```python
from build123d import *

# Parameters (mm, degrees)
F0_W      = 18
F0_H      = 20
F0_R      = 2.5
F0_W_2    = 31
F0_H_2    = 18
F0_H_3    = 2
F1_DEPTH  = 5
F2_DEPTH  = 14
F3_W      = 16
F3_H      = 7
F5_W      = 16
F5_H      = 7
F7_DEPTH  = 0.25
F4_W      = 16
F4_H      = 7
F6_W      = 16
F6_H      = 7
F8_DEPTH  = 0.25
F9_R      = 0.24999
F10_R     = 1
F11_W     = 20
F11_H     = 6
F12_DEPTH = 2
F13_SIZE  = 1


# Not quite as in the source:
# - a fillet or chamfer is up to 0.001 mm smaller than in the source, because OpenCascade refuses the exact size


with BuildPart() as f1:
    # F0 (on Top) → F1 (new body)
    with BuildSketch(Plane.XY):
        with Locations((-38.5, 0)):
            Rectangle(F0_W, F0_H)
        with Locations((-39.5, 0)):
            Circle(F0_R, mode=Mode.SUBTRACT)
        Polygon((-24.5, 10), (-29.5, 10), (-29.5, -10), (-24.5, -10), (-24.5, 8), align=None)
        with Locations((-9, -1)):
            Rectangle(F0_W_2, F0_H_2)
        Polygon((11.5, 10), (6.5, 10), (6.5, 8), (6.5, -10), (11.5, -10), (11.5, 8), align=None)
        Polygon((47.5, 10), (42.5, 10), (42.5, 8), (42.5, -10), (47.5, -10), align=None)
        with Locations((-9, 9)):
            Rectangle(F0_W_2, F0_H_3)
        with Locations((27, -1)):
            Rectangle(F0_W_2, F0_H_2)
        with Locations((27, 9)):
            Rectangle(F0_W_2, F0_H_3)
    extrude(amount=F1_DEPTH)

    # F0 (on Top) → F2 (join)
    with BuildSketch(Plane.XY):
        Polygon((-24.5, 10), (-29.5, 10), (-29.5, -10), (-24.5, -10), (-24.5, 8), align=None)
        Polygon((11.5, 10), (6.5, 10), (6.5, 8), (6.5, -10), (11.5, -10), (11.5, 8), align=None)
        Polygon((47.5, 10), (42.5, 10), (42.5, 8), (42.5, -10), (47.5, -10), align=None)
        with Locations((-9, 9)):
            Rectangle(F0_W_2, F0_H_3)
        with Locations((27, 9)):
            Rectangle(F0_W_2, F0_H_3)
    extrude(amount=F2_DEPTH)

    # F3 (on face) + F5 (on face) → F7 (join)
    with BuildSketch(Plane.YZ.offset(-24.5)):
        with Locations((-1, 9.5)):
            Rectangle(F3_W, F3_H)
    with BuildSketch(Plane.YZ.offset(11.5)):
        with Locations((-1, 9.5)):
            Rectangle(F5_W, F5_H)
    extrude(amount=F7_DEPTH)

    # F4 (on face) + F6 (on face) → F8 (join)
    with BuildSketch(Plane(origin=(6.5, 0, 0), x_dir=(0, -1, 0), z_dir=(-1, 0, 0))):
        with Locations((1, 9.5)):
            Rectangle(F4_W, F4_H)
    with BuildSketch(Plane(origin=(42.5, 0, 0), x_dir=(0, -1, 0), z_dir=(-1, 0, 0))):
        with Locations((1, 9.5)):
            Rectangle(F6_W, F6_H)
    extrude(amount=F8_DEPTH)

    # F9 (radius 0.25 in the source; OpenCascade refuses exactly that, so slightly less here)
    f9_edges = [f1.edges().sort_by_distance(p)[0] for p in [
        (-24.25, -1, 13),
        (-24.25, -9, 9.5),
        (-24.25, -1, 6),
        (-24.25, 7, 9.5),
        (6.25, 7, 9.5),
        (6.25, -1, 6),
        (6.25, -9, 9.5),
        (6.25, -1, 13),
        (11.75, -1, 13),
        (11.75, -9, 9.5),
        (11.75, -1, 6),
        (11.75, 7, 9.5),
        (42.25, -1, 13),
        (42.25, 7, 9.5),
        (42.25, -1, 6),
        (42.25, -9, 9.5),
    ]]
    fillet(f9_edges, radius=F9_R)

    # F10
    f10_edges = [f1.edges().sort_by_distance(p)[0] for p in [
        (-27, -10, 14),
        (9, -10, 14),
        (45, -10, 14),
        (9, 10, 14),
        (-47.5, -10, 2.5),
        (-47.5, 10, 2.5),
        (47.5, -10, 7),
        (47.5, 10, 7),
        (47.5, 0, 14),
        (-29.5, -10, 9.5),
        (-29.5, 10, 9.5),
    ]]
    fillet(f10_edges, radius=F10_R)

    # F11 (on face) → F12 (join)
    with BuildSketch(Plane.XY):
        with Locations((27.5, 0)):
            Rectangle(F11_W, F11_H)
    extrude(amount=-F12_DEPTH)

    # F13
    f13_edges = [f1.edges().sort_by_distance(p)[0] for p in [
        (27.5, -3, -2),
        (27.5, 3, -2),
    ]]
    chamfer(f13_edges, length=F13_SIZE)


solid = f1.part
```
Source: CAD feature listing. Evaluate the final solid. Frame: model axes, mm. A direction names the side the tool comes from. Give positions to 0.01 mm unless a question says otherwise; leave off trailing zeros. Loops run counter-clockwise (first coordinate to the right, second up) from the corner with the lowest first, then second, coordinate; pieces in that order, holes last. Notation, with made-up numbers: M 61.5,85.5 L 77.5,85.5 A13 cw 77.5,108.5 Z; hole C 2.25,-33 d1. An arc over 180 degrees is marked long. Put each result on its own line as item: value.
Q1. Section B-B (x = -16.5). Return the cut outline in (y, z), and give its area (3 significant figures).
Response values:
outline: M -10,0 L 10,0 L 10,13 A1 ccw 9,14 L 8,14 L 8,5 L -10,5 Z
area: 118 mm²
Q2. Pin query (flat end, axial travel): P1, Ø1, axis at y = 4.5, z = 9, coming from the -X side; P2, Ø1, axis at y = -1.5, z = -1.5, coming from the -X side; P3, Ø1, axis at x = 29.5, y = -3.5, coming from the +Z side; P4, Ø2, axis at y = 0, z = -0.5, coming from the +X side. Return the tip coordinate at first contact, or that it passes through.
Response values:
P1: stops at x = -29.5
P2: stops at x = 17.5
P3: stops at z = 5
P4: stops at x = 47.5
Q3. Section A-A (x = -39.5). Return the cut outline in (y, z), and give its area (3 significant figures).
Response values:
outline: M -10,0 L -2.5,0 L -2.5,5 L -10,5 Z; M 2.5,0 L 10,0 L 10,5 L 2.5,5 Z
area: 75.0 mm²
Q4. Mould query, pull axis X, two halves, no side actions, for faces 1 (the flat face through (6.25, -1, 10)), 2 (the flat face through (47.5, 0, 6)), 3 (the flat face through (1, 10, 6)), 4 (the flat face through (27, 8, 9)). Classes: released by +X, released by -X, zero draft, split by the parting line, or undercut.
Response values:
face 1: undercut
face 2: released by +X
face 3: zero draft
face 4: undercut
Q5. Line query: probe 1 along X at (y, z) = (7.5, 11.25); probe 2 along X at (y, z) = (-4, 9); probe 3 along Y at (x, z) = (-39.5, 2.85). Output: solid intervals per line, ascending. Write a range as [from, to].
Response values:
probe 1: x = [-29.5, -24.5], [6.5, 11.5], [42.5, 47.5]
probe 2: x = [-29.5, -24.25], [6.25, 11.75], [42.25, 47.5]
probe 3: y = [-10, -2.5], [2.5, 10]
Q6. Reachability of faces 5 (the flat face through (42.5, -0.3, 5.8)), 6 (the flat face through (-29.5, 0, 9)), 7 (the flat face through (17.5, 0, -1)), 8 (the flat face through (-24.25, -1, 10)) from +Z, -Z, +X, -X, +Y, -Y: full face, straight path, thin tool, end or side. Return the list, or none.
Response values:
face 5: none
face 6: +Z, -X, +Y, -Y
face 7: -Z, -X, +Y, -Y
face 8: +Z, -Y
